```python
from build123d import *

# Parameters (mm, degrees)
SKETCH1_W           = 70
SKETCH1_H           = 48
SKETCH1_W_2         = 43
SKETCH1_H_2         = 42.8
BOSS_EXTRUDE1_DEPTH = 4
SKETCH2_W           = 10.268328243
SKETCH2_H           = 48
SKETCH2_R           = 2.1
SKETCH2_W_2         = 10.814622491
BOSS_EXTRUDE2_DEPTH = 1.5
CHAMFER1_SIZE       = 6
FILLET1_R           = 2
SKETCH3_W           = 43
SKETCH3_H           = 7.264710946
CUT_EXTRUDE1_DEPTH  = 10
BOSS_EXTRUDE3_DEPTH = 45.8
BOSS_EXTRUDE4_DEPTH = 1.2
CUT_EXTRUDE2_DEPTH  = 50


with BuildPart() as part:
    # Sketch1 → Boss-Extrude1 (new body)
    with BuildSketch(Plane(origin=(0, 0, 789.620141885), x_dir=(-1, 0, 0), z_dir=(0, 0, -1))):
        with Locations((-51.439156386, -559.298939869)):
            Rectangle(SKETCH1_W, SKETCH1_H)
        with Locations((-51.439156386, -560.298939869)):
            Rectangle(SKETCH1_W_2, SKETCH1_H_2, mode=Mode.SUBTRACT)
        Polygon((-84.989156386, -558.249346414), (-84.989156386, -562.348533325), (-81.439156386, -564.398126781), (-77.889156386, -562.348533325), (-77.889156386, -558.249346414), (-81.439156386, -556.199752958), align=None, mode=Mode.SUBTRACT)
        Polygon((-17.889156386, -562.348533325), (-17.889156386, -558.249346414), (-21.439156386, -556.199752958), (-24.989156386, -558.249346414), (-24.989156386, -562.348533325), (-21.439156386, -564.398126781), align=None, mode=Mode.SUBTRACT)
    extrude(amount=BOSS_EXTRUDE1_DEPTH)

    # Sketch2 → Boss-Extrude2 (add)
    # profile 1 of 2: a face of its own
    with BuildSketch(Plane.XY.offset(789.620141885)):
        with Locations((21.573320508, -559.298939869)):
            Rectangle(SKETCH2_W, SKETCH2_H)
        with Locations((21.439156386, -560.298939869)):
            Circle(SKETCH2_R, mode=Mode.SUBTRACT)
    # profile 2 of 2: a face of its own
    with BuildSketch(Plane.XY.offset(789.620141885)):
        with Locations((81.03184514, -559.298939869)):
            Rectangle(SKETCH2_W_2, SKETCH2_H)
        with Locations((81.439156386, -560.298939869)):
            Circle(SKETCH2_R, mode=Mode.SUBTRACT)
    extrude(amount=-BOSS_EXTRUDE2_DEPTH)

    # Chamfer1
    chamfer1_edges = [part.edges().sort_by_distance(p)[0] for p in [
        (86.439156386, -535.298939869, 787.620141885),
        (16.439156386, -535.298939869, 787.620141885),
        (16.439156386, -583.298939869, 787.620141885),
        (86.439156386, -583.298939869, 787.620141885),
    ]]
    chamfer(chamfer1_edges, length=CHAMFER1_SIZE)

    # Fillet1
    fillet1_edges = [part.edges().sort_by_distance(p)[0] for p in [
        (72.939156386, -538.898939869, 787.620141885),
        (29.939156386, -538.898939869, 787.620141885),
    ]]
    fillet(fillet1_edges, radius=FILLET1_R)

    # Sketch3 → Cut-Extrude1 (cut)
    with BuildSketch(Plane(origin=(0, 0, 785.620141885), x_dir=(-1, 0, 0), z_dir=(0, 0, -1))):
        with Locations((-51.439156386, -585.331295342)):
            Rectangle(SKETCH3_W, SKETCH3_H)
    extrude(amount=-CUT_EXTRUDE1_DEPTH, mode=Mode.SUBTRACT)

    # Sketch4 → Boss-Extrude3 (add)
    with BuildSketch(Plane(origin=(0, 0, 785.620141885), x_dir=(-1, 0, 0), z_dir=(0, 0, -1))):
        Polygon((-86.439156386, -577.298939869), (-86.439156386, -541.298939869), (-80.439156386, -535.298939869), (-22.439156386, -535.298939869), (-16.439156386, -541.298939869), (-16.439156386, -577.298939869), (-17.939156386, -577.298939869), (-17.939156386, -541.920260213), (-23.06047673, -536.798939869), (-79.817836043, -536.798939869), (-84.939156386, -541.920260213), (-84.939156386, -577.298939869), align=None)
    extrude(amount=BOSS_EXTRUDE3_DEPTH)

    # Sketch5 → Boss-Extrude4 (add)
    with BuildSketch(Plane(origin=(0, 0, 739.820141885), x_dir=(-1, 0, 0), z_dir=(0, 0, -1))):
        Polygon((-86.439156386, -559.298939869), (-86.439156386, -541.298939869), (-80.439156386, -535.298939869), (-22.439156386, -535.298939869), (-16.439156386, -541.298939869), (-16.439156386, -559.298939869), (-16.439156386, -565.298939869), (-86.439156386, -565.298939869), align=None)
    extrude(amount=-BOSS_EXTRUDE4_DEPTH)

    # Sketch6 → Cut-Extrude2 (cut)
    with BuildSketch(Plane(origin=(0, 0, 785.620141885), x_dir=(-1, 0, 0), z_dir=(0, 0, -1))):
        Polygon((-17.939156386, -565.298939869), (-100.122525481, -565.298939869), (-100.122525481, -581.771183043), (-17.939156386, -581.771183043), (-3.612614588, -581.771183043), (-3.612614588, -565.298939869), align=None)
    extrude(amount=CUT_EXTRUDE2_DEPTH, mode=Mode.SUBTRACT)


solid = part.part
```
Build history of the part. All positions in model axes, mm. A direction names the side the tool comes from. Give positions to 0.01 mm unless a question says otherwise; leave off trailing zeros. Loops run counter-clockwise (first coordinate to the right, second up) from the corner with the lowest first, then second, coordinate; pieces in that order, holes last.
Item 1: Slice it at A-A, the plane y = -569. List the corners of the cut face in (x, z), and give its area (3 significant figures).
Answers follow:
outline: (16.44, 785.62) - (29.94, 785.62) - (29.94, 789.62) - (16.44, 789.62) - close; (72.94, 785.62) - (86.44, 785.62) - (86.44, 789.62) - (72.94, 789.62) - close
area: 108 mm2
Item 2: Pull direction Z, two halves, no side cores. Call faces 5 (the face through (51, -550, 739.82)), 6 (the face through (52, -535.299, 765)), 7 (the face through (79.64, -557.24, 786.89)): released by +Z, released by -Z, zero draft, split by the parting line, or undercut.
Answers follow:
face 5: released by -Z
face 6: zero draft
face 7: undercut
Item 3: Flat gauge pin, fed straight in: pin 1 (1 mm diameter, centred on x = 64.5, y = -561.5, fed in from +Z). Where does the tip first touch, or does it go through?
Answers follow:
pin 1: stops at z = 741.02
Item 4: Slice it at C-C, the plane y = -554. List the corners of the cut face in (x, z).
Answers follow:
outline: (16.44, 739.82) - (86.44, 739.82) - (86.44, 789.62) - (72.94, 789.62) - (72.94, 785.62) - (84.94, 785.62) - (84.94, 741.02) - (17.94, 741.02) - (17.94, 785.62) - (29.94, 785.62) - (29.94, 789.62) - (16.44, 789.62) - close
Item 5: Which spindle directions (+Z, -Z, +X, -X, +Y, -Y) get a long thin tool onto all of the face, cutting with end or side? Do faces 1 (the face through (17.939, -554, 764)), 2 (the face through (79.34, -560.21, 788.88)), 3 (the face through (77.889, -560, 787)), 4 (the face through (29.939, -562, 788)). Say none if no direction does.
Answers follow:
face 1: -Y
face 2: +Z
face 3: none
face 4: +Z, -Y
Item 6: Drill centre lines: line 1 (X direction, y = -544, z = 784); line 2 (Z direction, x = 77, y = -539.5); line 3 (Y direction, x = 45, z = 769). Where is each one in solid material? Low to high.
Answers follow:
line 1: x = 16.44 to 17.94, 84.94 to 86.44
line 2: z = 739.82 to 741.02, 785.62 to 789.62
line 3: y = -536.8 to -535.3
Item 7: Slice it at D-D, the plane z = 784. List the corners of the cut face in (x, y).
Answers follow:
outline: (16.44, -565.3) - (17.94, -565.3) - (17.94, -541.92) - (23.06, -536.8) - (79.82, -536.8) - (84.94, -541.92) - (84.94, -565.3) - (86.44, -565.3) - (86.44, -541.3) - (80.44, -535.3) - (22.44, -535.3) - (16.44, -541.3) - close
Item 8: Slice it at B-B, the plane x = 40.5. List the corners of the cut face in (y, z), and give its area (3 significant figures).
Answers follow:
outline: (-565.3, 739.82) - (-535.3, 739.82) - (-535.3, 789.62) - (-538.9, 789.62) - (-538.9, 785.62) - (-536.8, 785.62) - (-536.8, 741.02) - (-565.3, 741.02) - close
area: 117 mm2
